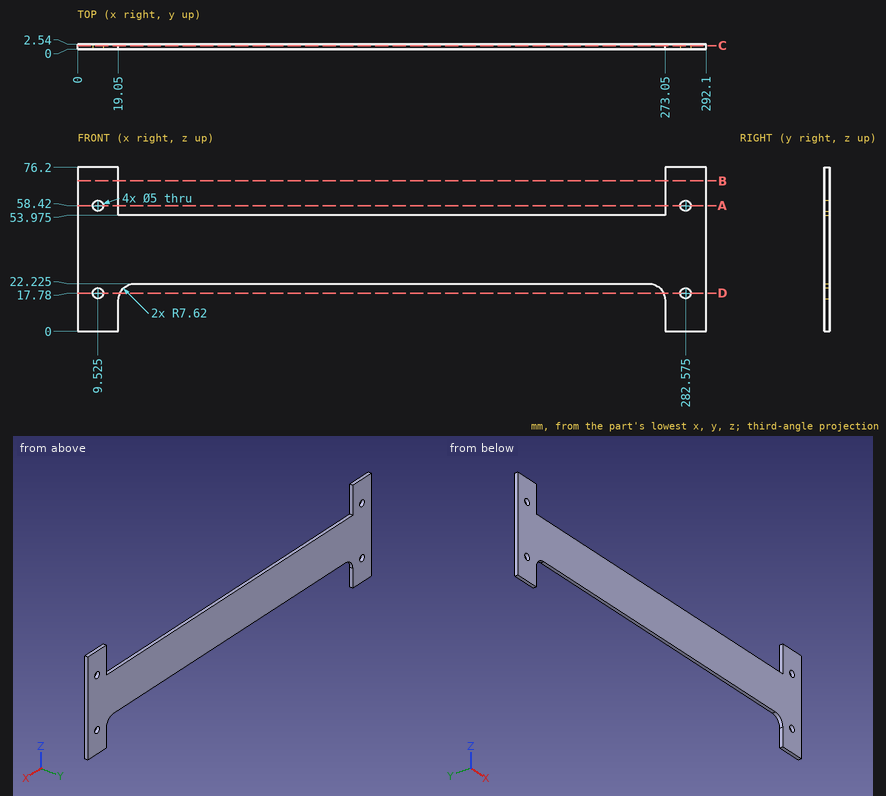
Verification items for this drawing (mm, ordinates from the low corner). Round coordinates to 2 decimals unless told otherwise and drop trailing zeros. Loops run counter-clockwise (first coordinate to the right, second up) from the corner with the lowest first, then second, coordinate; pieces in that order, holes last. Notation, with made-up numbers: (29, 7) - (50, 7) arc R27 ccw to (50, 45) - close; hole circle Ø1 at (4, 67.25). An arc over 180 degrees is marked (long way). Answer as CSV lines item,"result". Start each with the question number.
Item 1: Section check A-A (z = 58.42). Record the boundary of the cut face in (x, y) (3 decimals).
Item 2: Depth check by flat-ended pin: P1, Ø1, axis at x = 195.5, y = 0.5, coming from the -Z side (3 decimals). Enter the tip coordinate at first touch or a pass-through.
Item 3: Section check C-C (y = 1.75). Record the boundary of the cut face in (x, z) (3 decimals), and give its area (3 significant figures).
Item 4: Section check B-B (z = 70). Record the boundary of the cut face in (x, y).
Item 5: Section check D-D (z = 17.78). Record the boundary of the cut face in (x, y) (3 decimals).
Item 6: Scan lines: line 1 (X direction, y = 1.95, z = 58.42) (3 decimals); line 2 (X direction, y = 2.15, z = 66.5); line 3 (X direction, y = 1.5, z = 17.78) (3 decimals). Record each from-to range of solid material in increasing order. Write a range as [from, to].
Report:
1,outline,"(0, 0) - (7.025, 0) - (7.025, 2.54) - (0, 2.54) - close; (12.025, 0) - (19.05, 0) - (19.05, 2.54) - (12.025, 2.54) - close; (273.05, 0) - (280.075, 0) - (280.075, 2.54) - (273.05, 2.54) - close; (285.075, 0) - (292.1, 0) - (292.1, 2.54) - (285.075, 2.54) - close"
2,P1,"stops at z = 22.225"
3,outline,"(0, 0) - (19.05, 0) - (19.05, 14.605) arc R7.62 cw to (26.67, 22.225) - (265.43, 22.225) arc R7.62 cw to (273.05, 14.605) - (273.05, 0) - (292.1, 0) - (292.1, 76.2) - (273.05, 76.2) - (273.05, 53.975) - (19.05, 53.975) - (19.05, 76.2) - (0, 76.2) - close; hole circle Ø5 at (9.525, 17.78); hole circle Ø5 at (9.525, 58.42); hole circle Ø5 at (282.575, 17.78); hole circle Ø5 at (282.575, 58.42)"
3,area,"10,900 mm2"
4,outline,"(0, 0) - (19.05, 0) - (19.05, 2.54) - (0, 2.54) - close; (273.05, 0) - (292.1, 0) - (292.1, 2.54) - (273.05, 2.54) - close"
5,outline,"(0, 0) - (7.025, 0) - (7.025, 2.54) - (0, 2.54) - close; (12.025, 0) - (19.743, 0) - (19.743, 2.54) - (12.025, 2.54) - close; (272.357, 0) - (280.075, 0) - (280.075, 2.54) - (272.357, 2.54) - close; (285.075, 0) - (292.1, 0) - (292.1, 2.54) - (285.075, 2.54) - close"
6,line 1,"x = [0, 7.025], [12.025, 19.05], [273.05, 280.075], [285.075, 292.1]"
6,line 2,"x = [0, 19.05], [273.05, 292.1]"
6,line 3,"x = [0, 7.025], [12.025, 19.743], [272.357, 280.075], [285.075, 292.1]"
